from build123d import *

# Parameters (mm, degrees)
F0_W     = 355.6
F0_H     = 177.8
F1_DEPTH = 19.05
F3_DEPTH = 19.05


with BuildPart() as f1:
    # F0 (on Front) → F1 (new body)
    with BuildSketch(Plane.XZ):
        with Locations((177.8, 88.9)):
            Rectangle(F0_W, F0_H)
    extrude(amount=F1_DEPTH)

    # F2 (on Right) → F3 (cut)
    with BuildSketch(Plane.YZ):
        Polygon((0, 143.810647), (-12.7, 146.05), (-12.7, 107.95), (0, 110.189353), align=None)
        Polygon((0, 38.468058), (0, 72.089353), (-12.7, 74.328705), (-12.7, 36.228705), align=None)
    extrude(amount=F3_DEPTH, mode=Mode.SUBTRACT)


solid = f1.part
Check sheet for the modelled part. Datum: model origin and axes. Units: mm. A direction names the side the tool comes from. Give positions to 0.01 mm unless a question says otherwise; leave off trailing zeros. Loops run counter-clockwise (first coordinate to the right, second up) from the corner with the lowest first, then second, coordinate; pieces in that order, holes last. Notation, with made-up numbers: M -14,50 L 7,50 A28 cw 7,85 Z; hole C 37,14.5 d1. An arc over 180 degrees is marked long. Return JSON: item names as keys, results as strings. Group by question number.
1. Thickness scan on L1, parallel to X at y = -9.75, z = 44. Record the ranges inside material, lowest first.
2. Go/stop test with flat-tipped pins: pin 1 (21 mm diameter, centred on x = 6, z = 128.5, fed in from +Y); pin 2 (3 mm diameter, centred on y = -7, z = 60, fed in from -X). Record where each tip stops, or that it passes through.
3. Mould release check, pull along Y, two halves, no side actions. Record for faces 3 (the flat face through (9.392, -6.439, 109.054)), 4 (the flat face through (355.6, -9, 88)), 5 (the flat face through (9.392, -6.261, 144.915)), 6 (the flat face through (175, -19.05, 90)): released by +Y, released by -Y, zero draft, split by the parting line, or undercut.
4. Cross-section at A-A on z = 131. Record the boundary of the cut face in (x, y).
5. Tool access check on faces 1 (the flat face through (9.392, -6.439, 37.333)), 2 (the flat face through (175, 0, 90)). Record the directions out of +Z, -Z, +X, -X, +Y, -Y that give a thin tool (end or side, any length) a straight path to the whole face; none if there is none.
6. Cross-section at B-B on y = -5. Record the boundary of the cut face in (x, z), plus the area to 3 significant figures.
Return value:
{
 "1": {"L1": "19.05 to 355.6"},
 "2": {"pin 1": "y = -12.7", "pin 2": "x = 19.05"},
 "3": {"face 3": "undercut", "face 4": "zero draft", "face 5": "undercut", "face 6": "released by -Y"},
 "4": {"outline": "M 0,-19.05 L 355.6,-19.05 L 355.6,0 L 19.05,0 L 19.05,-12.7 L 0,-12.7 Z"},
 "5": {"face 1": "-X", "face 2": "+Z, -Z, +X, -X, +Y"},
 "6": {"outline": "M 0,0 L 355.6,0 L 355.6,177.8 L 0,177.8 L 0,144.69 L 19.05,144.69 L 19.05,109.31 L 0,109.31 L 0,72.97 L 19.05,72.97 L 19.05,37.59 L 0,37.59 Z", "area": "61,900 mm^2"}
}
